Could you check a few things on this model? Use its own coordinates, in mm. Face numbers are marked on the shaded views. A direction names the side the tool comes from. Round coordinates to 2 decimals unless told otherwise and drop trailing zeros. Write each loop counter-clockwise with the first axis right and the second up, starting at its lowest first coordinate (ties: lowest second). Pieces come first, ordered by that corner, then holes. Notation, with made-up numbers: (18.5, 39.5) - (38.5, 39.5) arc R26 ccw to (38.5, 59.5) - close; hole circle Ø3 at (61, 22). An arc over 180 degrees is marked (long way). Put each result on its own line as item: value.
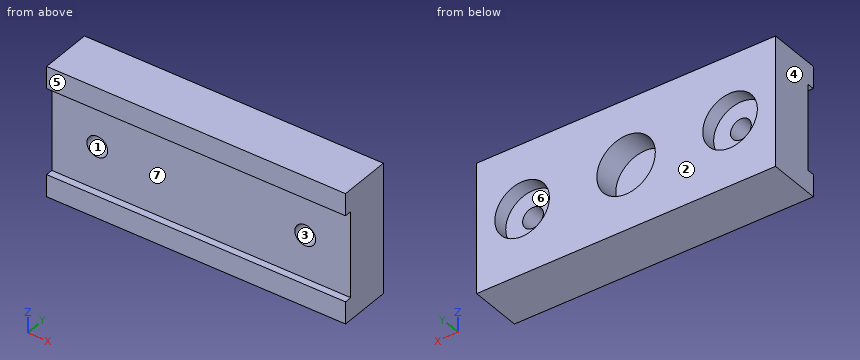
from build123d import *

# Parameters (mm, degrees)
SKETCH1_W                                        = 46
SKETCH1_H                                        = 20
BOSS_EXTRUDE1_DEPTH                              = 8
SKETCH3_R                                        = 4.5
CUT_EXTRUDE2_DEPTH                               = 4
CUT_EXTRUDE3_REACH                               = 49.749
CBORE_FOR_M3_HEX_HEAD_MACHINE_SCREW1_D           = 3.2
CBORE_FOR_M3_HEX_HEAD_MACHINE_SCREW1_CBORE_D     = 8.4
CBORE_FOR_M3_HEX_HEAD_MACHINE_SCREW1_CBORE_DEPTH = 2.3


with BuildPart() as part:
    # Sketch1 → Boss-Extrude1 (new body)
    with BuildSketch(Plane(origin=(0, 0, 0), x_dir=(1, 0, 0), z_dir=(0, 1, 0))):
        Rectangle(SKETCH1_W, SKETCH1_H)
    extrude(amount=BOSS_EXTRUDE1_DEPTH)

    # Sketch3 → Cut-Extrude2 (cut)
    with BuildSketch(Plane(origin=(0, 8, 0), x_dir=(1, 0, 0), z_dir=(0, 1, 0))):
        with Locations(Location((0, 0, 0), (0, 0, 270))):
            Circle(SKETCH3_R)
    extrude(amount=-CUT_EXTRUDE2_DEPTH, mode=Mode.SUBTRACT)

    # Sketch8 → Cut-Extrude3 (cut, up to next)
    with BuildSketch(Plane.ZY.offset(23), mode=Mode.PRIVATE) as cut_extrude3_sk1:
        Polygon((0, 0), (-6.6, 0), (-6.6, 1.1), (6.6, 1.1), (6.6, 0), align=None)
    cut_extrude3_tool1 = extrude(cut_extrude3_sk1.sketch, amount=-CUT_EXTRUDE3_REACH, mode=Mode.PRIVATE) & part.part
    add(cut_extrude3_tool1.solids().sort_by_distance((-23, 0.55, 0))[0], mode=Mode.SUBTRACT)

    # CBORE for M3 Hex Head Machine Screw1 (through all)
    with Locations(Plane(origin=(0, 8, 0), x_dir=(1, 0, 0), z_dir=(0, 1, 0))):
        with Locations((-16, 0), (16, 0)):
            CounterBoreHole(CBORE_FOR_M3_HEX_HEAD_MACHINE_SCREW1_D / 2, CBORE_FOR_M3_HEX_HEAD_MACHINE_SCREW1_CBORE_D / 2, CBORE_FOR_M3_HEX_HEAD_MACHINE_SCREW1_CBORE_DEPTH)


solid = part.part
(1) Please list where these lines run through material, in increasing order: probe 1 along Z at (x, y) = (-16, 7.15); probe 2 along Z at (x, y) = (16.5, 0.5); probe 3 along Y at (x, z) = (-8.5, -3.5). Write a range as from..to.
Values found:
probe 1: z = -10..-4.2, 4.2..10
probe 2: z = -10..-6.6, 6.6..10
probe 3: y = 1.1..8
(2) Imagine slicing it at D-D, the plane x = 0. List the corners of the cut face in (y, z) for me.
Values found:
outline: (0, -10) - (8, -10) - (8, -4.5) - (4, -4.5) - (4, 4.5) - (8, 4.5) - (8, 10) - (0, 10) - (0, 6.6) - (1.1, 6.6) - (1.1, -6.6) - (0, -6.6) - close
(3) Imagine slicing it at C-C, the plane y = 6.5. List the corners of the cut face in (x, z) for me.
Values found:
outline: (-23, -10) - (23, -10) - (23, 10) - (-23, 10) - close; hole circle Ø8.4 at (-16, 0); hole circle Ø9 at (0, 0); hole circle Ø8.4 at (16, 0)
(4) For the marked faces 5, 6 and 7, which set-ups out of +Z, -Z, +X, -X, +Y, -Y let a thin tool reach every point of the face, with its end or its side?
Values found:
face 5: +Z, -Z, +X, -X, -Y
face 6: +Y
face 7: +X, -X, -Y
(5) If we mould it in two halves opening along X, with no side actions, what happens to the marked faces 1, 2, 3 and 4? For each: pulls with the +X half, pulls with the -X half, needs draft (parallel to the pull), parting line crosses it, or undercut.
Values found:
face 1: undercut
face 2: needs draft
face 3: undercut
face 4: pulls with the -X half
(6) Imagine slicing it at A-A, the plane z = 0. List the corners of the cut face in (x, y) for me.
Values found:
outline: (-23, 1.1) - (-17.6, 1.1) - (-17.6, 5.7) - (-20.2, 5.7) - (-20.2, 8) - (-23, 8) - close; (-14.4, 1.1) - (14.4, 1.1) - (14.4, 5.7) - (11.8, 5.7) - (11.8, 8) - (4.5, 8) - (4.5, 4) - (-4.5, 4) - (-4.5, 8) - (-11.8, 8) - (-11.8, 5.7) - (-14.4, 5.7) - close; (17.6, 1.1) - (23, 1.1) - (23, 8) - (20.2, 8) - (20.2, 5.7) - (17.6, 5.7) - close
(7) Imagine slicing it at B-B, the plane x = 16. List the corners of the cut face in (y, z) for me, then the cut area to 3 significant figures.
Values found:
outline: (0, -10) - (8, -10) - (8, -4.2) - (5.7, -4.2) - (5.7, -1.6) - (1.1, -1.6) - (1.1, -6.6) - (0, -6.6) - close; (0, 6.6) - (1.1, 6.6) - (1.1, 1.6) - (5.7, 1.6) - (5.7, 4.2) - (8, 4.2) - (8, 10) - (0, 10) - close
area: 111 mm^2
(8) I'm going to push flat-ended pins straight in: pin 1 (4 mm diameter, centred on x = -0.5, z = 3, fed in from -Y); pin 2 (2.5 mm diameter, centred on x = 1, z = -1, fed in from +Y); pin 3 (4 mm diameter, centred on x = 14.5, z = 0, fed in from +Y). Where does each tip first touch, or does it pass through?
Values found:
pin 1: stops at y = 1.1
pin 2: stops at y = 4
pin 3: stops at y = 5.7
